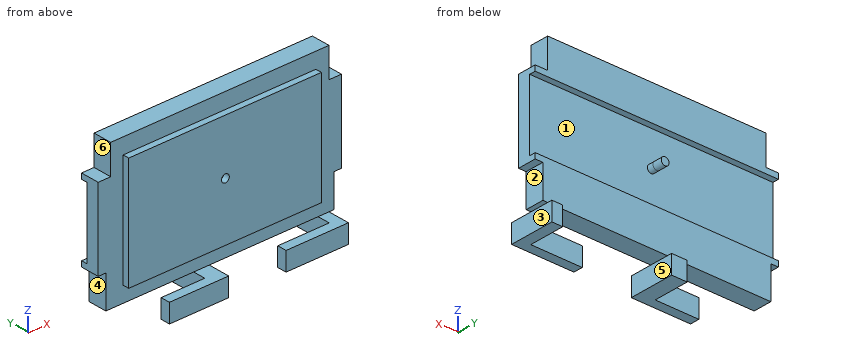
Autodesk Inventor part; units mm, degrees
ref_plane "YZ Plane" through (0, 0, 0) normal (1, 0, 0) x (0, 1, 0)
ref_plane "XZ Plane" through (0, 0, 0) normal (0, 1, 0) x (-1, 0, 0)
ref_plane "XY Plane" through (0, 0, 0) normal (0, 0, 1) x (1, 0, 0)
sketch "Sketch1" plane through (0, 0, 0) normal (0, 1, 0) x (-1, 0, 0)
  line L0 (-36.5556, -23.5) -> (36.5556, -23.5)
  line L1 (35, 22.5) -> (-35, 22.5)
  line L2 (-36.5556, -23.5) -> (35, 22.5) construction
  line L3 (36.5556, -23.5) -> (-35, 22.5) construction
  line L4 (-39, 0) -> (-39, -11)
  line L5 (-39, -11) -> (-39, 11)
  line L6 (39, -11) -> (39, 11)
  line L7 (-39, -11) -> (-39, -13)
  line L8 (-39, -13) -> (-36.5556, -13)
  line L9 (-39, 11) -> (-39, 13)
  line L10 (-39, 13) -> (-35, 13)
  line L11 (39, -11) -> (39, -13)
  line L12 (39, -13) -> (36.5556, -13)
  line L13 (39, 11) -> (39, 13)
  line L14 (39, 13) -> (35, 13)
  line L15 (-30.788, 17.5) -> (31, 17.5)
  line L16 (31, 17.5) -> (31, -18.5)
  line L17 (31, -18.5) -> (-30.788, -18.5)
  line L18 (-30.788, -18.5) -> (-30.788, 17.5)
  line L19 (-30.788, 17.5) -> (31, -18.5) construction
  line L20 (31, 17.5) -> (-30.788, -18.5) construction
  line L21 (36.5556, -23.5) -> (36.5556, -13)
  line L22 (35, 13) -> (35, 22.5)
  line L23 (-35, 22.5) -> (-35, 13)
  line L24 (-36.5556, -13) -> (-36.5556, -23.5)
  circle A0 centre (0, 0) radius 1.25
  dimension "d133" = 2.5
  dimension "d169" = 36
  dimension "d170" = 4
  dimension "d171" = 5
  dimension "d180" = 46
extrude "Extrusion39" add sketch "Sketch1" along normal blind 6 contours L24 L8 L7 L4 L5 L9 L10 L23 L1 L22 L14 L13 L6 L11 L12 L21 L0
extrude "Extrusion40" add sketch "Sketch1" against normal blind 2 contours L15 L16 L17 L18
extrude "Extrusion41" add sketch "Sketch1" along normal blind 6 contours L15 L16 L17 L18
extrude "Extrusion42" add sketch "Sketch1" along normal blind 9 contours A0
sketch "Sketch30" plane through (0, 6, 0) normal (0, 1, 0) x (1, 0, 0)
  line L0 (-39, -11.25) -> (39, -11.25)
  line L1 (39, -11.25) -> (39, 11.25)
  line L2 (39, 11.25) -> (-39, 11.25)
  line L3 (-39, 11.25) -> (-39, -11.25)
  circle A0 centre (0, 0) radius 1.25
  line L4 (-39, -11.25) -> (39, 11.25) construction
  line L5 (39, -11.25) -> (-39, 11.25) construction
  dimension "d142" = 78
  dimension "d143" = 22.5
extrude "Extrusion43" cut sketch "Sketch30" against normal blind 2
sketch "Sketch31" plane through (36.5556, 0, -23.5) normal (0, 0, -1) x (-1, 0, 0)
  line L0 (67.5556, 0) -> (5.7676, 0)
  line L1 (67.5556, 0) -> (67.5556, -2)
  line L2 (64.95, 0) -> (44.95, 0)
  line L3 (44.95, 0) -> (44.95, 7.5)
  line L4 (39.95, 7.5) -> (39.95, -7)
  line L5 (39.95, -7) -> (58.95, -7)
  line L6 (58.95, -7) -> (58.95, -4)
  line L7 (58.95, -4) -> (44.95, -4)
  line L8 (44.95, -4) -> (44.95, 0)
  line L9 (75.5556, 4) -> (-2.4444, 4)
  line L10 (5.05, 0) -> (5.05, 4)
  line L11 (1.5556, 0) -> (1.5556, 6)
  line L12 (71.5556, 0) -> (1.5556, 0)
  line L13 (1.5556, 0) -> (1.5556, -7)
  line L14 (1.5556, -7) -> (21.5556, -7)
  line L15 (21.5556, -7) -> (21.5556, -4)
  line L16 (21.5556, -4) -> (5.05, -4)
  line L17 (5.7676, 0) -> (5.7676, -2)
  line L18 (5.05, -4) -> (5.05, 0)
  line L19 (44.95, 7.5) -> (39.95, 7.5)
  line L20 (5.05, 4) -> (5.05, 7.5)
  line L21 (5.05, 7.5) -> (1.5556, 7.5)
  line L22 (1.5556, 7.5) -> (1.5556, -7)
  point P0 (36.5556, 0)
  point P1 (-2.4444, 4)
  point P2 (66, 0)
  point P3 (4.212, 0)
  dimension "d152" = 5
  dimension "d157" = 20
  dimension "d163" = 4
  dimension "d164" = 4
  dimension "d187" = 3
  dimension "d188" = 3
extrude "Extrusion51" cut sketch "Sketch31" along normal blind 10 contours L18 L16 L15 L14 L13 L12
extrude "Extrusion52" cut sketch "Sketch31" along normal blind 10 contours L12 L11 L9 L10 | L9 L11 L22 L21 L20
extrude "Extrusion54" add sketch "Sketch31" along normal blind 6 contours L12 L11 L9 L10 | L18 L16 L15 L14 L13 L12 | L9 L11 L22 L21 L20
extrude "Extrusion55" add sketch "Sketch31" along normal blind 6 contours L8 L7 L6 L5 L4 L0 | L0 L4 L9 L3 | L9 L4 L19 L3
equation "\"d187\" = d188"
properties part number "kotelon yläosa"
The model under review builds one solid part; all positions refer to its coordinate system, in mm. Face numbers are marked on the shaded views. A direction names the side the tool comes from. Coordinates: 2 decimals unless noted, no trailing zeros. Loops run counter-clockwise (first coordinate to the right, second up) from the corner with the lowest first, then second, coordinate; pieces in that order, holes last. Notation, with made-up numbers: M -2,81.25 L 46,81.25 A4 cw 46,85.25 Z; hole C 56.5,-19.5 d6. An arc over 180 degrees is marked long. Put each result on its own line as item: value. Start each with the question number.
Q1. Add section C-C (x = -6). Write out the cut boundary in (y, z), and give its area (3 significant figures).
Q2. Add section B-B (z = 14). Write out the cut boundary in (x, y), and give its area (3 significant figures).
Q3. Wall thickness on line 1 (X direction, y = -5, z = -26.5); line 2 (Z direction, x = 0, y = -0.6); line 3 (Z direction, x = -5.5, y = 5.5): over which ranges is each line inside the solid? List them lowest first.
Q4. Add section A-A (x = -15). Write out the cut boundary in (y, z).
Q5. Clearance check with flat-ended pins moving along their axes: pin 1 (0.7 mm diameter, centred on x = -37, y = 4, fed in from -Z); pin 2 (2 mm diameter, centred on x = 0, z = 0, fed in from -Y); pin 3 (2.5 mm diameter, centred on x = 37.5, y = 2, fed in from -Z). State where each tip first meets the part, or that it passes through.
Q6. For the marked faces 3, 4, 5 and 6, list the 3-axis set-ups (+Z, -Z, +X, -X, +Y, -Y) from which the entire face can be reached by the end or side of a thin tool; tool diameter is ignored.
Q7. The part is to be moulded in two halves that separate along Z. For the marked faces 1 and 2, say which applies: +Z half, -Z half, draft (parallel to the pull), parting line (faces both ways), or undercut.
Q8. Add section D-D (z = 8.5). Write out the cut boundary in (x, y).
Answers:
1. outline: M -7,-29.5 L 7.5,-29.5 L 7.5,-23.5 L 6,-23.5 L 6,-11.25 L 4,-11.25 L 4,11.25 L 6,11.25 L 6,22.5 L 0,22.5 L 0,17.5 L -2,17.5 L -2,-18.5 L 0,-18.5 L 0,-23.5 L -7,-23.5 Z
1. area: 390 mm^2
2. outline: M -35,0 L -31,0 L -31,-2 L 30.79,-2 L 30.79,0 L 35,0 L 35,6 L -35,6 Z
2. area: 544 mm^2
3. line 1: x = -22.39 to -3.39, 15 to 35
3. line 2: z = -18.5 to -1.25, 1.25 to 17.5
3. line 3: z = -29.5 to -11.25, 11.25 to 22.5
4. outline: M -7,-29.5 L -4,-29.5 L -4,-23.5 L -7,-23.5 Z; M -2,-18.5 L 0,-18.5 L 0,-23.5 L 6,-23.5 L 6,-11.25 L 4,-11.25 L 4,11.25 L 6,11.25 L 6,22.5 L 0,22.5 L 0,17.5 L -2,17.5 Z
5. pin 1: stops at z = -13
5. pin 2: stops at y = 0
5. pin 3: stops at z = -23.5
6. face 3: -Z, +X, +Y, -Y
6. face 4: -Z, -X, +Y, -Y
6. face 5: -Z, +Y, -Y
6. face 6: +Z, -X, +Y, -Y
7. face 1: undercut
7. face 2: draft
8. outline: M -39,0 L -31,0 L -31,-2 L 30.79,-2 L 30.79,0 L 39,0 L 39,4 L -39,4 Z
